```python
from build123d import *

# Parameters (mm, degrees)
SKETCH1_R           = 50.8
SKETCH1_R_2         = 49.2125
BOSS_EXTRUDE1_DEPTH = 1016
CUT_EXTRUDE1_START  = 127
SKETCH2_W           = 2.9972
SKETCH2_H           = 38.1
CUT_EXTRUDE1_DEPTH  = 50.0126


with BuildPart() as part:
    # Sketch1 → Boss-Extrude1 (new body)
    with BuildSketch(Plane.XY):
        Circle(SKETCH1_R)
        Circle(SKETCH1_R_2, mode=Mode.SUBTRACT)
    extrude(amount=BOSS_EXTRUDE1_DEPTH)

    # Sketch2 → Cut-Extrude1 (cut)
    with BuildSketch(Plane.XY.offset(CUT_EXTRUDE1_START)):
        Polygon((25.020238518, -16.17587567), (26.518838518, -13.58022433), (59.514406402, -32.63022433), (58.015806402, -35.22587567), align=None)
        with Locations((0, 49.2125)):
            Rectangle(SKETCH2_W, SKETCH2_H)
        Polygon((-26.870791242, -13.37702433), (-25.372191242, -15.97267567), (-58.367759126, -35.02267567), (-59.866359126, -32.42702433), align=None)
    extrude(amount=-CUT_EXTRUDE1_DEPTH, mode=Mode.SUBTRACT)


solid = part.part
```
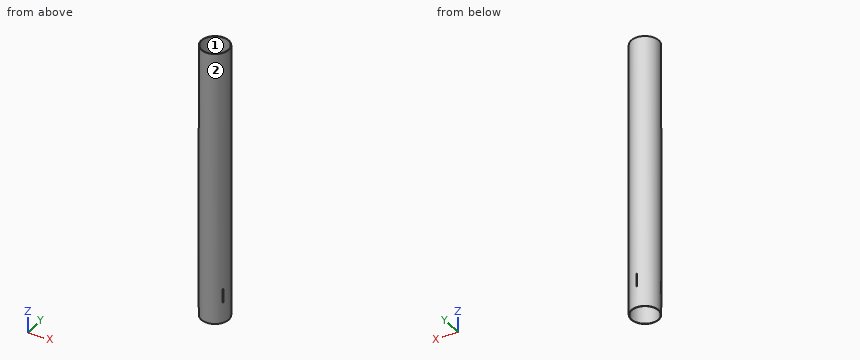
Work out the finished part from the listing and answer in its coordinate system (mm). Face numbers are marked on the shaded views. Give positions to 0.01 mm unless a question says otherwise; leave off trailing zeros. Write each loop counter-clockwise with the first axis right and the second up, starting at its lowest first coordinate (ties: lowest second). Pieces come first, ordered by that corner, then holes. Notation, with made-up numbers: (62, -13.75) -> (81, -13.75) arc R10 ccw to (81, 4.25) -> close; hole circle Ø8 at (-35, -38.75). An arc over 180 degrees is marked (long way). Write each question's results on one line, items separated by ' | '.
1. Find section C-C on z = 795.5. Determine the outline of the cut face in (x, y) (1 decimal), and give its area (3 significant figures).
Data:
outline: circle Ø101.6 at (0, 0); hole circle Ø98.4 at (0, 0) | area: 499 mm^2
2. Each of these flat-tipped pins is pushed along its axis until it touches: pin 1 Ø1 at (x, z) = (18, 169.5) entering from +Y; pin 2 Ø12 at (x, z) = (27, 676) entering from -Y; pin 3 Ø6 at (x, z) = (-23.5, 848) entering from +Y; pin 4 Ø5 at (x, y) = (-22.5, 39.5) entering from +Z. Where does it stop, or does it pass through?
Data:
pin 1: y = 47.69 | pin 2: y = -46.26 | pin 3: y = 46.48 | pin 4: through
3. Straight lines are drawn through the part: L1, parallel to Y at x = 0, z = 495; L2, parallel to Y at x = 3.5, z = 441; L3, parallel to X at y = -2, z = 139.5. For each, find the intervals that lie inside material, in ascending order.
Data:
L1: -50.8 to -49.21, 49.21 to 50.8 | L2: -50.68 to -49.09, 49.09 to 50.68 | L3: -50.76 to -49.17, 49.17 to 50.76
4. Determine the mould class of the marked faces 1 and 2 for opening direction X: +X half, -X half, draft (parallel to the pull), parting line (faces both ways), or undercut.
Data:
face 1: undercut | face 2: parting line
5. Find section B-B on x = -22. Determine the outline of the cut face in (y, z).
Data:
outline: (-45.79, 0) -> (-44.02, 0) -> (-44.02, 1016) -> (-45.79, 1016) -> close; (44.02, 0) -> (45.79, 0) -> (45.79, 1016) -> (44.02, 1016) -> close
6. Find section A-A on y = 0. Determine the outline of the cut face in (x, z).
Data:
outline: (-50.8, 0) -> (-49.21, 0) -> (-49.21, 1016) -> (-50.8, 1016) -> close; (49.21, 0) -> (50.8, 0) -> (50.8, 1016) -> (49.21, 1016) -> close
